Model file for the job. Use its own axes, mm. Face numbers are marked on the shaded views. A direction names the side the tool comes from. Round coordinates to 2 decimals unless told otherwise and drop trailing zeros. Order: outer loops, then holes, each group sorted by start corner. A loop starts at its lowest first (then second) coordinate and runs counter-clockwise, first axis right, second up. Notation, with made-up numbers: (10, 35.5) - (60, 35.5) arc R8 ccw to (60, 39.5) - close; hole circle Ø5 at (11.5, 58.25). An arc over 180 degrees is marked (long way). Write item = value, one per line.
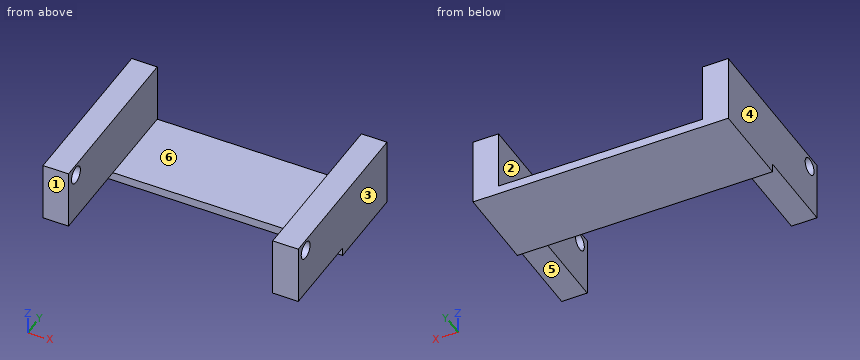
Autodesk Inventor part; units mm, degrees
ref_plane "YZ Plane" through (0, 0, 0) normal (1, 0, 0) x (0, 1, 0)
ref_plane "XZ Plane" through (0, 0, 0) normal (0, 1, 0) x (-1, 0, 0)
ref_plane "作業平面1" through (0, 0, -20) normal (0, 0, 1) x (1, 0, 0)
sketch "スケッチ1" plane through (0, 0, -20) normal (0, 0, 1) x (1, 0, 0)
  line L0 (-45, 55) -> (45, 55)
  line L1 (45, 55) -> (45, 25)
  line L2 (45, 25) -> (-45, 25)
  line L3 (-45, 25) -> (-45, 55)
  line L4 (0, 66) -> (0, -11)
  line L5 (-63, 0) -> (63, 0)
  point P0 (0, 0)
  dimension "d1" = 90
  dimension "d2" = 30
  dimension "d3" = 55
extrude "押し出し1" add sketch "スケッチ1" along normal blind 3
sketch "スケッチ2" plane through (0, 0, -17) normal (0, 0, 1) x (1, 0, 0)
  line L0 (45, 55) -> (-45, 55)
  line L1 (45, 55) -> (36, 55)
  line L2 (36, 55) -> (36, -5)
  line L3 (36, -5) -> (45, -5)
  line L4 (45, -5) -> (45, 55)
  line L5 (-45, 55) -> (-45, 25)
  line L6 (-45, 55) -> (-36, 55)
  line L7 (-36, 55) -> (-36, -5)
  line L8 (-36, -5) -> (-45, -5)
  line L9 (-45, -5) -> (-45, 55)
  point P0 (0, 0)
  dimension "d6" = 9
  dimension "d7" = 60
  dimension "d8" = 9
extrude "押し出し2" add sketch "スケッチ2" along normal blind 21
sketch "スケッチ3" plane through (0, 0, 0) normal (1, 0, 0) x (0, 1, 0)
  circle A0 centre (0, 0) radius 3
  dimension "d11" = 6
extrude "押し出し3" cut sketch "スケッチ3" along normal up to surface (90 mm away) from surface at -45
properties part number "vacuum_cup_base"
1) Cut at D-D (z = 0). Write the cut outline in (x, y).
Conclusion:
outline = (-45, -5) - (-36, -5) - (-36, -3) - (-45, -3) - close; (-45, 3) - (-36, 3) - (-36, 55) - (-45, 55) - close; (36, -5) - (45, -5) - (45, -3) - (36, -3) - close; (36, 3) - (45, 3) - (45, 55) - (36, 55) - close
2) Mould opens along X. For the marked faces 1, 2 and 3 say: +X half, -X half, draft (parallel to the pull), parting line (faces both ways), or undercut.
Conclusion:
face_1 = draft
face_2 = undercut
face_3 = +X half
3) Wall check: line 1 along X through (y, z) = (16, -6.25); line 2 along Y through (x, z) = (39.25, 0); line 3 along Z through (x, y) = (-40, 0). Give the ranges that are in metal, low to high.
Conclusion:
line_1 = -45 to -36, 36 to 45
line_2 = -5 to -3, 3 to 55
line_3 = -17 to -3, 3 to 4
4) Cut at C-C (y = 0). Write the cut outline in (x, z).
Conclusion:
outline = (-45, -17) - (-36, -17) - (-36, -3) - (-45, -3) - close; (-45, 3) - (-36, 3) - (-36, 4) - (-45, 4) - close; (36, -17) - (45, -17) - (45, -3) - (36, -3) - close; (36, 3) - (45, 3) - (45, 4) - (36, 4) - close
5) Flat gauge pins, fed straight in: pin 1 Ø1.5 at (x, z) = (19.5, -19) entering from -Y; pin 2 Ø7 at (x, y) = (-40, 4) entering from -Z; pin 3 Ø9 at (x, y) = (-13, 41) entering from +Z. Where does each tip first touch, or does it go through?
Conclusion:
pin_1 = 25
pin_2 = -17
pin_3 = -17
6) Cut at B-B (z = -13). Write the cut outline in (x, y), and give its area (3 significant figures).
Conclusion:
outline = (-45, -5) - (-36, -5) - (-36, 55) - (-45, 55) - close; (36, -5) - (45, -5) - (45, 55) - (36, 55) - close
area = 1,080 mm^2
7) Cut at A-A (y = 19.5). Write the cut outline in (x, z), and give its area (3 significant figures).
Conclusion:
outline = (-45, -17) - (-36, -17) - (-36, 4) - (-45, 4) - close; (36, -17) - (45, -17) - (45, 4) - (36, 4) - close
area = 378 mm^2
8) 3-axis set-ups, long thin cutter, end or side, ignore diameter. For the marked faces 4, 5 and 6: which of +Z, -Z, +X, -X, +Y, -Y reach the whole face in a straight line?
Conclusion:
face_4 = +Z, -Z, -X, +Y, -Y
face_5 = -Z, +X, -X, -Y
face_6 = +Z, +Y, -Y
